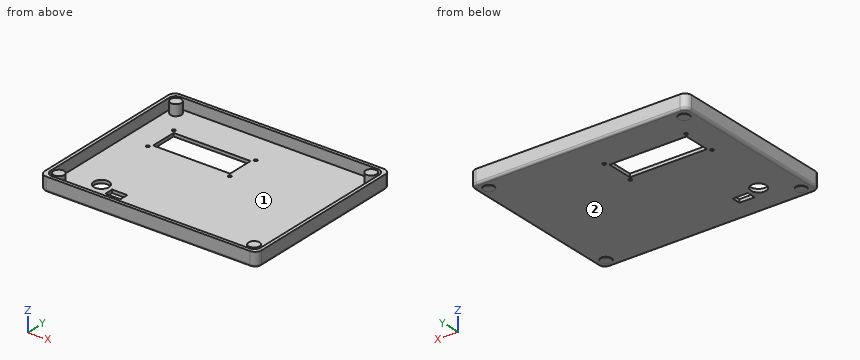
from build123d import *

# Parameters (mm, degrees)
BOSS_EXTRU_1_DEPTH      = 3
BOSS_EXTRU_2_START      = 10
BOSS_EXTRU_2_DEPTH      = 10
ESQUISSE2_R             = 5
BOSS_EXTRU_3_DEPTH      = 10
CONG_1_R                = 2
BOSS_EXTRU_4_START      = -3.5
ESQUISSE2_2_R           = 5
BOSS_EXTRU_4_DEPTH      = 3.5
ESQUISSE3_R             = 1.5
ESQUISSE3_W             = 71
ESQUISSE3_H             = 24.5
ENL_V_MAT_EXTRU_1_DEPTH = 3.5
ESQUISSE4_R             = 7
ESQUISSE4_W             = 14
ESQUISSE4_H             = 8
ENL_V_MAT_EXTRU_2_DEPTH = 10


with BuildPart() as part:
    # Esquisse1 → Boss.-Extru.1 (new body)
    # profile 1 of 2: a face of its own
    with BuildSketch(Plane.XY):
        with BuildLine():
            ThreePointArc((-100, 74), (-98.242640687, 78.242640687), (-94, 80))
            Line((-94, 80), (94, 80))
            ThreePointArc((94, 80), (98.242640687, 78.242640687), (100, 74))
            Line((100, 74), (100, -74))
            ThreePointArc((100, -74), (98.242640687, -78.242640687), (94, -80))
            Line((94, -80), (-94, -80))
            ThreePointArc((-94, -80), (-98.242640687, -78.242640687), (-100, -74))
            Line((-100, -74), (-100, 74))
        make_face()
        with BuildLine():
            Line((-97, -71), (-97, 71))
            ThreePointArc((-97, 71), (-95.242640687, 75.242640687), (-91, 77))
            Line((-91, 77), (91, 77))
            ThreePointArc((91, 77), (95.242640687, 75.242640687), (97, 71))
            Line((97, 71), (97, -71))
            ThreePointArc((97, -71), (95.242640687, -75.242640687), (91, -77))
            Line((91, -77), (-91, -77))
            ThreePointArc((-91, -77), (-95.242640687, -75.242640687), (-97, -71))
        make_face(mode=Mode.SUBTRACT)
    # profile 2 of 2: a face of its own
    with BuildSketch(Plane.XY):
        with BuildLine():
            ThreePointArc((-97, 71), (-95.242640687, 75.242640687), (-91, 77))
            Line((-91, 77), (91, 77))
            ThreePointArc((91, 77), (95.242640687, 75.242640687), (97, 71))
            Line((97, 71), (97, -71))
            ThreePointArc((97, -71), (95.242640687, -75.242640687), (91, -77))
            Line((91, -77), (-91, -77))
            ThreePointArc((-91, -77), (-95.242640687, -75.242640687), (-97, -71))
            Line((-97, -71), (-97, 71))
        make_face()
    extrude(amount=-BOSS_EXTRU_1_DEPTH)

    # Esquisse1_3 → Boss.-Extru.2 (add)
    with BuildSketch(Plane.XY.offset(BOSS_EXTRU_2_START)):
        with BuildLine():
            Line((-94, -80), (94, -80))
            ThreePointArc((94, -80), (98.242640687, -78.242640687), (100, -74))
            Line((100, -74), (100, 74))
            ThreePointArc((100, 74), (98.242640687, 78.242640687), (94, 80))
            Line((94, 80), (-94, 80))
            ThreePointArc((-94, 80), (-98.242640687, 78.242640687), (-100, 74))
            Line((-100, 74), (-100, -74))
            ThreePointArc((-100, -74), (-98.242640687, -78.242640687), (-94, -80))
        make_face()
        with BuildLine():
            Line((-91, -77), (91, -77))
            ThreePointArc((91, -77), (95.242640687, -75.242640687), (97, -71))
            Line((97, -71), (97, 71))
            ThreePointArc((97, 71), (95.242640687, 75.242640687), (91, 77))
            Line((91, 77), (-91, 77))
            ThreePointArc((-91, 77), (-95.242640687, 75.242640687), (-97, 71))
            Line((-97, 71), (-97, -71))
            ThreePointArc((-97, -71), (-95.242640687, -75.242640687), (-91, -77))
        make_face(mode=Mode.SUBTRACT)
    extrude(amount=-BOSS_EXTRU_2_DEPTH)

    # Esquisse2 → Boss.-Extru.3 (add)
    with BuildSketch(Plane.XY):
        with Locations((-90, 70)):
            Circle(ESQUISSE2_R)
        with Locations((90, 70)):
            Circle(ESQUISSE2_R)
        with Locations((90, -70)):
            Circle(ESQUISSE2_R)
        with Locations((-90, -70)):
            Circle(ESQUISSE2_R)
    extrude(amount=BOSS_EXTRU_3_DEPTH)

    # Cong_1
    cong_1_edges = [part.edges().sort_by_distance(p)[0] for p in [
        (-100, 0, -3),
        (-98.242640687, -78.242640687, -3),
        (0, -80, -3),
        (98.242640687, -78.242640687, -3),
        (100, 0, -3),
        (98.242640687, 78.242640687, -3),
        (0, 80, -3),
        (-98.242640687, 78.242640687, -3),
    ]]
    fillet(cong_1_edges, radius=CONG_1_R)

    # Esquisse2_2 → Boss.-Extru.4 (add)
    with BuildSketch(Plane.XY.offset(BOSS_EXTRU_4_START)):
        with Locations((-90, 70)):
            Circle(ESQUISSE2_2_R)
        with Locations((90, 70)):
            Circle(ESQUISSE2_2_R)
        with Locations((90, -70)):
            Circle(ESQUISSE2_2_R)
        with Locations((-90, -70)):
            Circle(ESQUISSE2_2_R)
    extrude(amount=BOSS_EXTRU_4_DEPTH)

    # Esquisse3 → Enl_v. mat.-Extru.1 (cut)
    with BuildSketch(Plane(origin=(0, 0, -3), x_dir=(-1, 0, 0), z_dir=(0, 0, -1))):
        with Locations((-0.6, 48)):
            Circle(ESQUISSE3_R)
        with Locations((-0.6, 17)):
            Circle(ESQUISSE3_R)
        with Locations((75, 17)):
            Circle(ESQUISSE3_R)
        with Locations((75, 48)):
            Circle(ESQUISSE3_R)
        with Locations((37.2, 32.5)):
            Rectangle(ESQUISSE3_W, ESQUISSE3_H)
    extrude(amount=-ENL_V_MAT_EXTRU_1_DEPTH, mode=Mode.SUBTRACT)

    # Esquisse4 → Enl_v. mat.-Extru.2 (cut)
    with BuildSketch(Plane(origin=(0, 0, -3), x_dir=(-1, 0, 0), z_dir=(0, 0, -1))):
        with Locations((66, -50.25)):
            Circle(ESQUISSE4_R)
        with Locations((48, -55.75)):
            Rectangle(ESQUISSE4_W, ESQUISSE4_H)
    extrude(amount=-ENL_V_MAT_EXTRU_2_DEPTH, mode=Mode.SUBTRACT)


solid = part.part
Build history of the part. All positions in model axes, mm. Face numbers are marked on the shaded views. A direction names the side the tool comes from. Give positions to 0.01 mm unless a question says otherwise; leave off trailing zeros. Write each loop counter-clockwise with the first axis right and the second up, starting at its lowest first coordinate (ties: lowest second). Pieces come first, ordered by that corner, then holes. Notation, with made-up numbers: (14.5, 47) - (35.5, 47) arc R12 ccw to (35.5, 69) - close; hole circle Ø8 at (51, 40). An arc over 180 degrees is marked (long way). Use one line per item in the form item = value. Start each with the question number.
1. 3-axis set-ups, long thin cutter, end or side, ignore diameter. For the marked faces 1 and 2: which of +Z, -Z, +X, -X, +Y, -Y reach the whole face in a straight line?
2. Drop flat-ended pins along their axis: pin 1 Ø2.5 at (x, z) = (-51, -2) entering from -Y; pin 2 Ø8 at (x, y) = (8.5, 36) entering from -Z; pin 3 Ø3.5 at (x, y) = (0.6, 48) entering from +Z; pin 4 Ø1.5 at (x, z) = (-51, -2) entering from +Y. Give the stop position or say it passes through.
3. Band-saw the part on A-A on x = -66. Write the cut outline in (y, z).
4. Band-saw the part on C-C on x = 47.5. Write the cut outline in (y, z), plus the area to 3 significant figures.
5. Band-saw the part on B-B on y = -36. Write the cut outline in (x, z).
6. Probe line 1 (Y direction, x = -8, z = 7.5); line 2 (X direction, y = 9, z = 5); line 3 (Y direction, x = -23.5, z = -0.25). List the from-to ranges inside material, lowest first. Write a range as [from, to].
Conclusion:
q1.face_1 = +Z
q1.face_2 = -Z
q2.pin_1 = -80
q2.pin_2 = -3
q2.pin_3 = 0
q2.pin_4 = 79.98
q3.outline = (-80, -1) arc R2 ccw to (-78, -3) - (-57.25, -3) - (-57.25, 0) - (-77, 0) - (-77, 10) - (-80, 10) - close; (-43.25, -3) - (20.25, -3) - (20.25, 0) - (-43.25, 0) - close; (44.75, -3) - (78, -3) arc R2 ccw to (80, -1) - (80, 10) - (77, 10) - (77, 0) - (44.75, 0) - close
q4.outline = (-80, -1) arc R2 ccw to (-78, -3) - (78, -3) arc R2 ccw to (80, -1) - (80, 10) - (77, 10) - (77, 0) - (-77, 0) - (-77, 10) - (-80, 10) - close
q4.area = 538 mm²
q5.outline = (-100, -1) arc R2 ccw to (-98, -3) - (98, -3) arc R2 ccw to (100, -1) - (100, 10) - (97, 10) - (97, 0) - (-97, 0) - (-97, 10) - (-100, 10) - close
q6.line_1 = [-80, -77], [77, 80]
q6.line_2 = [-100, -97], [97, 100]
q6.line_3 = [-80, 20.25], [44.75, 80]
